Job drawing, mm, ordinate dimensions from the low corner. One solid piece. A direction names the side the tool comes from. Round coordinates to 2 decimals unless told otherwise and drop trailing zeros. Loops run counter-clockwise (first coordinate to the right, second up) from the corner with the lowest first, then second, coordinate; pieces in that order, holes last.
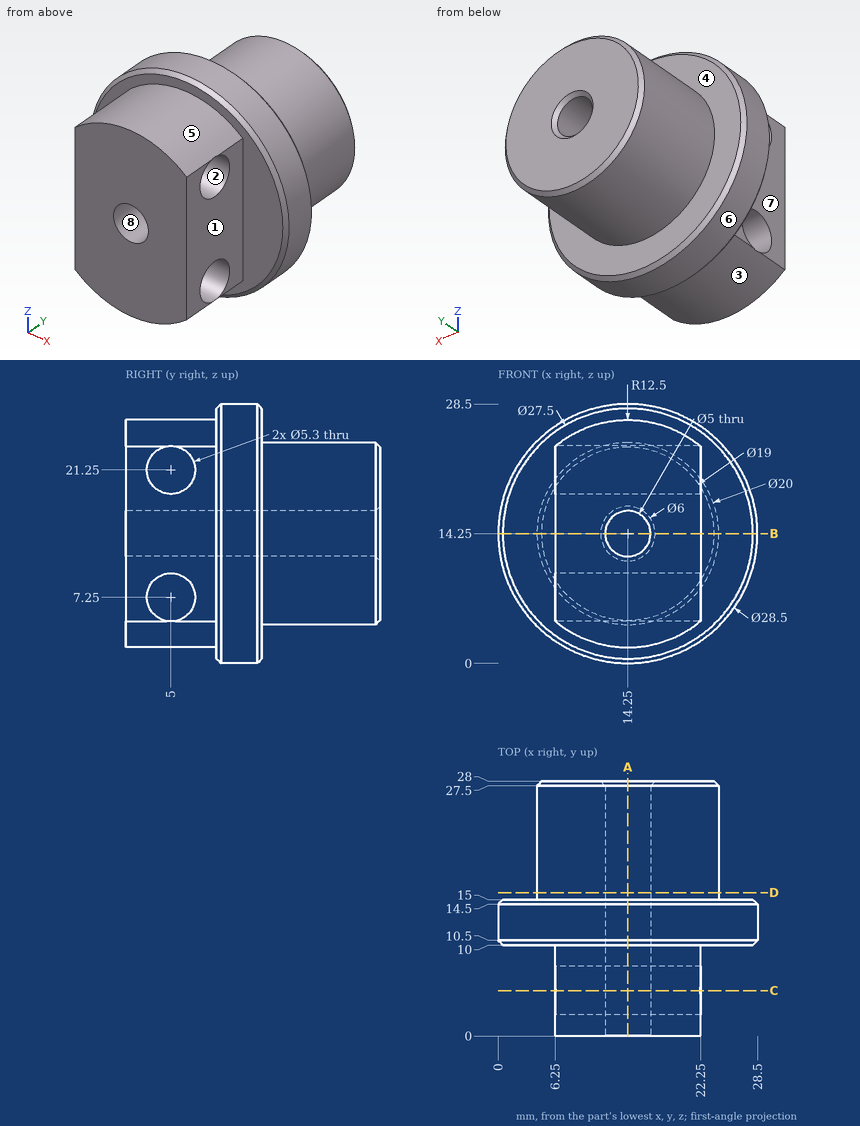
Item 1: Flat gauge pins, fed straight in: P1, Ø4, axis at y = 19.5, z = 3.5, coming from the -X side; P2, Ø1.5, axis at x = 25.5, y = 9, coming from the -Z side; P3, Ø2, axis at x = 23, z = 23.5, coming from the +Y side; P4, Ø5, axis at y = 5.5, z = 11, coming from the -X side. Where does each tip first touch, or does it go through?
Answers follow:
P1: stops at x = 9.41
P2: passes through
P3: stops at y = 15
P4: stops at x = 6.25
Item 2: Probe line 1 (X direction, y = 8.5, z = 14.25); line 2 (Y direction, x = 19, z = 7.25); line 3 (Z direction, x = 15.75, y = 3). List the from-to ranges inside material, lowest first.
Answers follow:
line 1: x = 6.25 to 11.75, 16.75 to 22.25
line 2: y = 0 to 2.35, 7.65 to 28
line 3: z = 1.84 to 5.51, 8.99 to 12.25, 16.25 to 19.51, 22.99 to 26.66
Item 3: Cut at A-A, the plane x = 14.25. Give the cut face in (y, z), plus the area to 3 significant figures.
Answers follow:
outline: (0, 1.75) - (10, 1.75) - (10, 0.5) - (10.5, 0) - (14.5, 0) - (15, 0.5) - (15, 4.25) - (27.5, 4.25) - (28, 4.75) - (28, 11.25) - (27.5, 11.75) - (0, 11.75) - close; (0, 16.75) - (27.5, 16.75) - (28, 17.25) - (28, 23.75) - (27.5, 24.25) - (15, 24.25) - (15, 28) - (14.5, 28.5) - (10.5, 28.5) - (10, 28) - (10, 26.75) - (0, 26.75) - close; hole circle Ø5.3 at (5, 7.25); hole circle Ø5.3 at (5, 21.25)
area: 467 mm2
Item 4: Cut at D-D, the plane y = 15.75. Give the cut face in (x, z).
Answers follow:
outline: circle Ø20 at (14.25, 14.25); hole circle Ø5 at (14.25, 14.25)
Item 5: Cut at B-B, the plane z = 14.25. Give the cut face in (x, y).
Answers follow:
outline: (0, 10.5) - (0.5, 10) - (6.25, 10) - (6.25, 0) - (11.75, 0) - (11.75, 27.5) - (11.25, 28) - (4.75, 28) - (4.25, 27.5) - (4.25, 15) - (0.5, 15) - (0, 14.5) - close; (16.75, 0) - (22.25, 0) - (22.25, 10) - (28, 10) - (28.5, 10.5) - (28.5, 14.5) - (28, 15) - (24.25, 15) - (24.25, 27.5) - (23.75, 28) - (17.25, 28) - (16.75, 27.5) - close
Item 6: Two-plate mould, pull along Z, no slides. Class the marked faces 6, 7 and 8: released by +Z, released by -Z, zero draft, split by the parting line, or undercut.
Answers follow:
face 6: split by the parting line
face 7: zero draft
face 8: undercut
Item 7: 3-axis set-ups, long thin cutter, end or side, ignore diameter. For the marked faces 1, 2, 3, 4 and 5: which of +Z, -Z, +X, -X, +Y, -Y reach the whole face in a straight line?
Answers follow:
face 1: +Z, -Z, +X, -Y
face 2: +X, -X
face 3: -Z, -Y
face 4: +Y
face 5: +Z, -Y
Item 8: Cut at C-C, the plane y = 5. Give the cut face in (x, z).
Answers follow:
outline: (6.25, 9.9) - (22.25, 9.9) - (22.25, 18.6) - (6.25, 18.6) - close; (6.3, 4.6) arc R12.5 ccw to (22.2, 4.6) - close; (6.3, 23.9) - (22.2, 23.9) arc R12.5 ccw to start; hole circle Ø5 at (14.25, 14.25)
